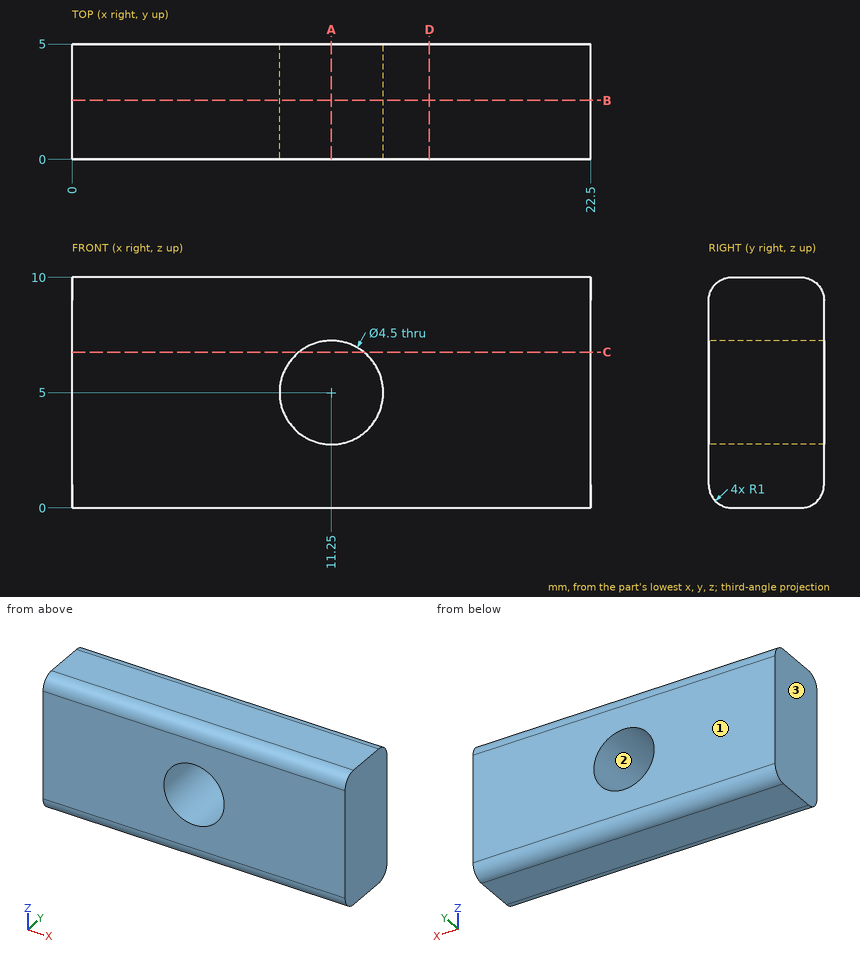
For this review, use the dimensioned drawing (mm, ordinates from the lowest corner) and the shaded views. Round coordinates to 2 decimals unless told otherwise and drop trailing zeros. Order: outer loops, then holes, each group sorted by start corner. A loop starts at its lowest first (then second) coordinate and runs counter-clockwise, first axis right, second up. Notation, with made-up numbers: M 22.25,-3 L 64.25,-3 A28 cw 64.25,26 Z; hole C -9.5,36.5 d11. An arc over 180 degrees is marked long. Use a Markdown table: item, result. Add a question column.
Item 1: Add section B-B, the plane y = 2.55. Give the boundary of the cut face in (x, z).
Item 2: Add section C-C, the plane z = 6.75. Give the boundary of the cut face in (x, y).
Item 3: Add section D-D, the plane x = 15.5. Give the boundary of the cut face in (y, z).
Item 4: To check wall thickness, follow line 1 along Z through (x, y) = (11.25, 3.4); line 2 along X through (y, z) = (0.7, 4); line 3 along X through (y, z) = (2.5, 3.75). State the ranges of each line that lie inside material, in increasing order.
Item 5: Mouldability with a two-part tool opening along X and no side actions: class the marked faces 1, 2 and 3 as released by +X, released by -X, zero draft, split by the parting line, or undercut.
Item 6: Add section A-A, the plane x = 11.25. Give the boundary of the cut face in (y, z), then the cut area to 3 significant figures.
Geometry results:
| question | item | result |
|---|---|---|
| 1 | outline | M 0,0 L 22.5,0 L 22.5,10 L 0,10 Z; hole C 11.25,5 d4.5 |
| 2 | outline | M 0,0 L 9.84,0 L 9.84,5 L 0,5 Z; M 12.66,0 L 22.5,0 L 22.5,5 L 12.66,5 Z |
| 3 | outline | M 0,1 A1 ccw 1,0 L 4,0 A1 ccw 5,1 L 5,9 A1 ccw 4,10 L 1,10 A1 ccw 0,9 Z |
| 4 | line 1 | z = 0 to 2.75, 7.25 to 10 |
| 4 | line 2 | x = 0 to 9.23, 13.27 to 22.5 |
| 4 | line 3 | x = 0 to 9.38, 13.12 to 22.5 |
| 5 | face 1 | zero draft |
| 5 | face 2 | undercut |
| 5 | face 3 | released by -X |
| 6 | outline | M 0,1 A1 ccw 1,0 L 4,0 A1 ccw 5,1 L 5,2.75 L 0,2.75 Z; M 0,7.25 L 5,7.25 L 5,9 A1 ccw 4,10 L 1,10 A1 ccw 0,9 Z |
| 6 | area | 26.6 mm² |
